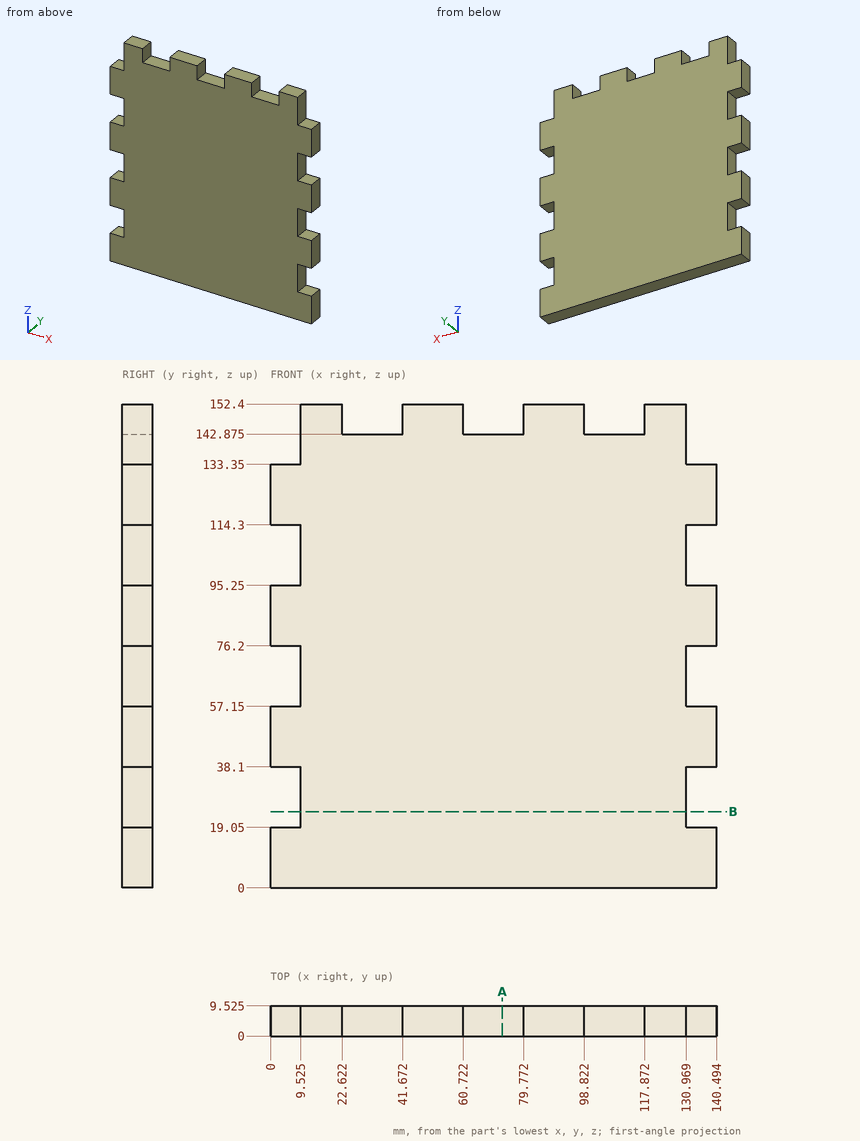
Drawing for the job (mm, zero at the part's lowest x, y, z). Round coordinates to 2 decimals unless told otherwise and drop trailing zeros. Write each loop counter-clockwise with the first axis right and the second up, starting at its lowest first coordinate (ties: lowest second). Pieces come first, ordered by that corner, then holes. Notation, with made-up numbers: (-11, 57.5) - (45, 57.5) arc R20 cw to (45, 90.5) - close; hole circle Ø3 at (51.25, 42.5). An arc over 180 degrees is marked (long way). Return JSON: item names as keys, results as strings. Group by question number.
Item 1: Band-saw the part on B-B on z = 24. List the corners of the cut face in (x, y) (1 decimal).
Item 2: Band-saw the part on A-A on x = 73. List the corners of the cut face in (y, z) (1 decimal).
Item 3: Probe probe 1 along Z at (x, y) = (105, 7.75) (1 decimal); probe 2 along X at (y, z) = (2.5, 97) (1 decimal). List the from-to ranges inside material, lowest first.
Item 4: Flat gauge pins, fed straight in: pin 1 Ø3 at (y, z) = (5.5, 148.5) entering from +X; pin 2 Ø3 at (x, y) = (4.5, 5) entering from +Z; pin 3 Ø5 at (y, z) = (4, 109.5) entering from -X (3 decimals). Where does each tip first touch, or does it go through?
Resolved:
{
 "1": {"outline": "(9.5, 0) - (131, 0) - (131, 9.5) - (9.5, 9.5) - close"},
 "2": {"outline": "(0, 0) - (9.5, 0) - (9.5, 142.9) - (0, 142.9) - close"},
 "3": {"probe 1": "z = 0 to 142.9", "probe 2": "x = 9.5 to 131"},
 "4": {"pin 1": "stops at x = 130.97", "pin 2": "stops at z = 133.35", "pin 3": "stops at x = 9.525"}
}
